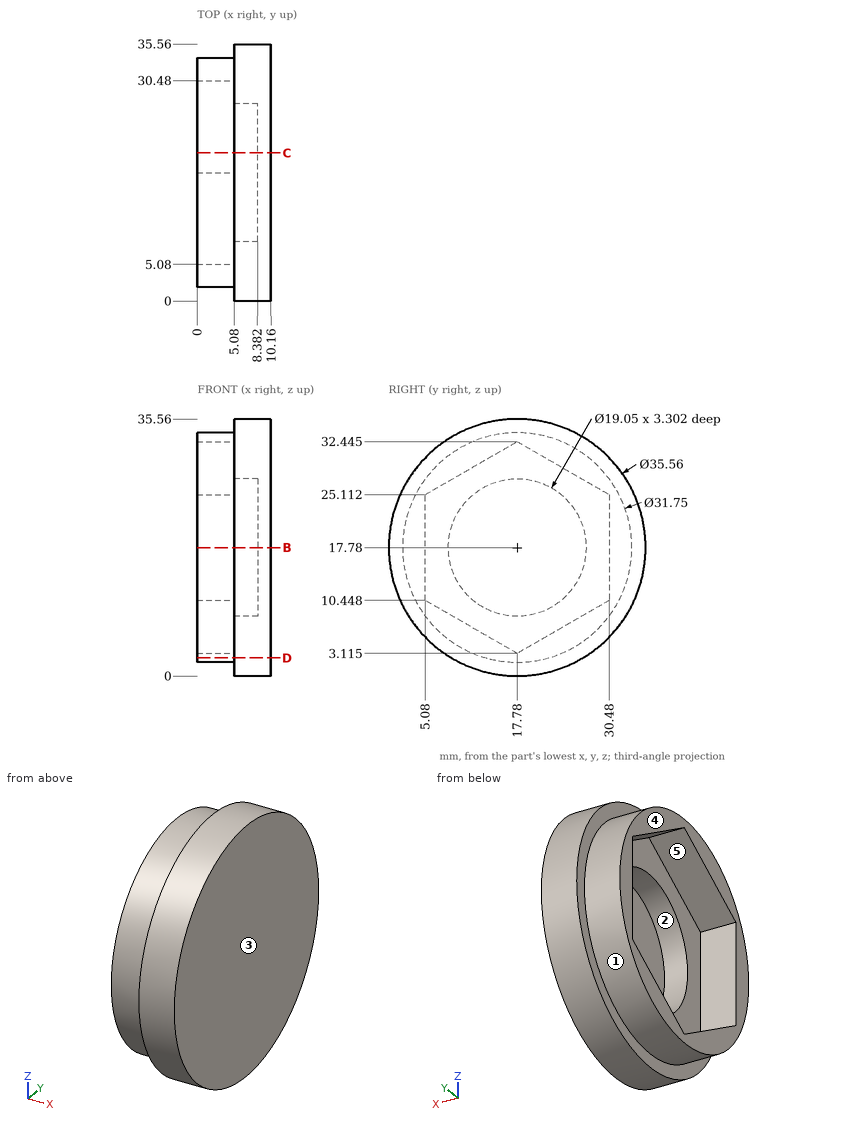
Can you work these out from the drawing? Everything is in mm from the part's minimum corner. A direction names the side the tool comes from. Coordinates: 2 decimals unless noted, no trailing zeros. Loops run counter-clockwise (first coordinate to the right, second up) from the corner with the lowest first, then second, coordinate; pieces in that order, holes last. Notation, with made-up numbers: M 55.25,-11.75 L 107.25,-11.75 A34 ccw 107.25,18.25 Z; hole C 56,12.5 d3. An arc over 180 degrees is marked long. One line per item, written item: value.
1. Thinking about a two-plate mould opening in Y: for the marked faces 1, 2 and 3, which applies, +Y half, -Y half, draft (parallel to the pull), parting line (faces both ways), or undercut?
Geometry says:
face 1: parting line
face 2: undercut
face 3: draft
2. Will these pins go through, and if not, where does the flat tip stop? pin 1 Ø1 at (y, z) = (19.5, 22.5) entering from -X; pin 2 Ø1 at (x, z) = (8, 13.5) entering from +Y; pin 3 Ø1 at (x, z) = (7.5, 25) entering from +Y.
Geometry says:
pin 1: stops at x = 8.38
pin 2: stops at y = 35.15
pin 3: stops at y = 34.24
3. Imagine slicing it at D-D (z = 2.5). List the corners of the cut face in (x, y) for me (1 decimal).
Geometry says:
outline: M 0,13.5 L 5.1,13.5 L 5.1,8.7 L 10.2,8.7 L 10.2,26.9 L 5.1,26.9 L 5.1,22.1 L 0,22.1 Z
4. On a 3-axis mill with a long thin cutter (end or side, diameter ignored), from which of +Z, -Z, +X, -X, +Y, -Y can I reach the whole of each face in a straight line? I mean the marked faces 4 and 5. Say none if no direction works.
Geometry says:
face 4: +Z, -Z, -X, +Y, -Y
face 5: -X
5. Imagine slicing it at C-C (y = 20.5). List the corners of the cut face in (x, z) for me (1 decimal), and give its area (3 significant figures).
Geometry says:
outline: M 0,2.1 L 5.1,2.1 L 5.1,0.2 L 10.2,0.2 L 10.2,35.4 L 5.1,35.4 L 5.1,33.4 L 0,33.4 L 0,30.9 L 5.1,30.9 L 5.1,26.9 L 8.4,26.9 L 8.4,8.7 L 5.1,8.7 L 5.1,4.7 L 0,4.7 Z
area: 144 mm2
6. Imagine slicing it at B-B (z = 17.78). List the corners of the cut face in (x, y) for me (1 decimal).
Geometry says:
outline: M 0,1.9 L 5.1,1.9 L 5.1,0 L 10.2,0 L 10.2,35.6 L 5.1,35.6 L 5.1,33.7 L 0,33.7 L 0,30.5 L 5.1,30.5 L 5.1,27.3 L 8.4,27.3 L 8.4,8.3 L 5.1,8.3 L 5.1,5.1 L 0,5.1 Z
7. Please list where these lines run through material, in increasing order: probe 1 along Z at (x, y) = (7.5, 17.78) (1 decimal); probe 2 along X at (y, z) = (21, 7); probe 3 along X at (y, z) = (19.5, 20).
Geometry says:
probe 1: z = 0 to 8.3, 27.3 to 35.6
probe 2: x = 5.08 to 10.16
probe 3: x = 8.38 to 10.16
